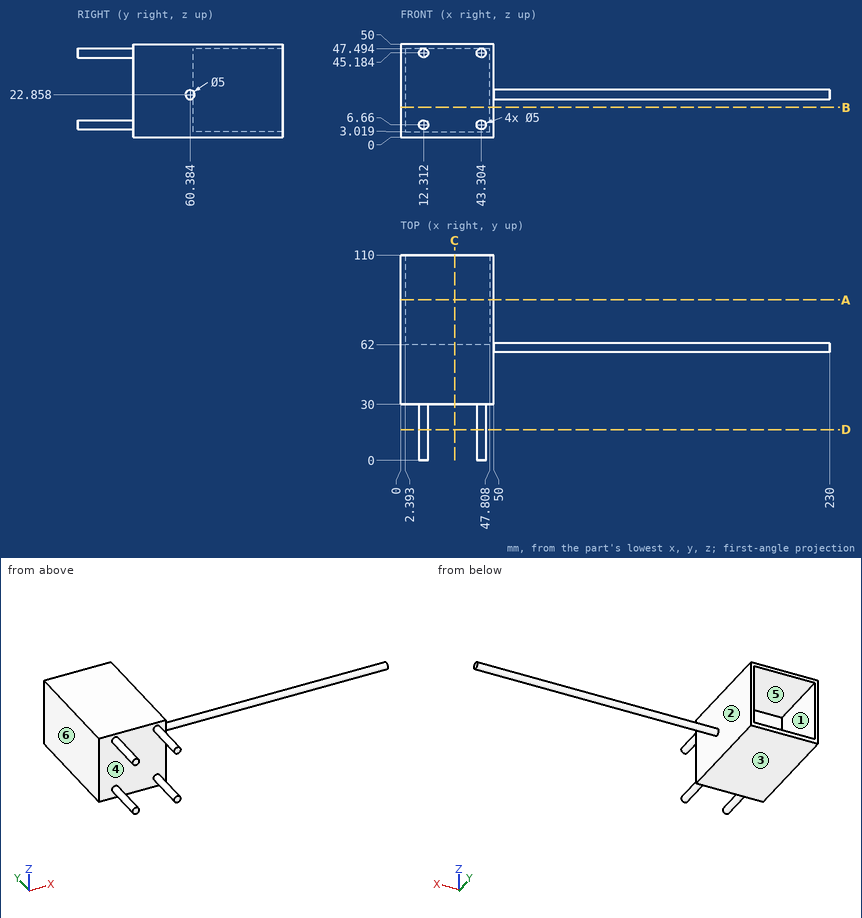
Study the drawing (mm; zero at the part's minimum x, y, z) and answer. A direction names the side the tool comes from. Round coordinates to 2 decimals unless told otherwise and drop trailing zeros. Write each loop counter-clockwise with the first axis right and the second up, starting at its lowest first coordinate (ties: lowest second). Pieces come first, ordered by that corner, then holes. Notation, with made-up numbers: (17.25, -32) -> (69.25, -32) arc R12 cw to (69.25, -17) -> close; hole circle Ø2 at (2.25, 72.25). An arc over 180 degrees is marked (long way). Answer as CSV lines item,"result". Start each with the question number.
(1) The part is cut by section C-C, the plane x = 29. Give the vertices of the cut face in (y, z) (1 decimal).
(2) Each of these flat-tipped pins is pushed along its axis until it touches: pin 1 (4 mm diameter, centred on x = 172.5, z = 21, fed in from -Y); pin 2 (13.5 mm diameter, centred on x = 22.5, y = 84, fed in from -Z); pin 3 (10 mm diameter, centred on y = 12.5, z = 5.5, fed in from +X) (1 decimal); pin 4 (22 mm diameter, centred on x = 33.5, z = 33.5, fed in from +Y). Where does it stop, or does it pass through?
(3) The part is cut by section A-A, the plane y = 86. Give the vertices of the cut face in (x, z) (1 decimal).
(4) A tool of negligible diameter and unlimited length cuts with its end or side. For the marked faces 4, 5 and 6, from which of +Z, -Z, +X, -X, +Y, -Y can it reach the whole face along a straight path? Write none if from no direction.
(5) The part is cut by section D-D, the plane y = 16.5. Give the vertices of the cut face in (x, z) (1 decimal).
(6) The mould has two halves that part along X. Classify the marked faces 1, 2 and 3: +X half, -X half, draft (parallel to the pull), parting line (faces both ways), or undercut.
(7) The part is cut by section B-B, the plane z = 16. Give the vertices of the cut face in (x, y).
(8) Find the intervals of material crossed by probe 1 along X at (y, z) = (98, 43); probe 2 along Z at (x, y) = (31.5, 98.5) (1 decimal); probe 3 along Y at (x, z) = (20, 18), in increasing order.
Output values:
1,outline,"(30, 0) -> (110, 0) -> (110, 3) -> (62, 3) -> (62, 47.5) -> (110, 47.5) -> (110, 50) -> (30, 50) -> close"
2,pin 1,"stops at y = 57.88"
2,pin 2,"stops at z = 0"
2,pin 3,"stops at x = 45.8"
2,pin 4,"stops at y = 62"
3,outline,"(0, 0) -> (50, 0) -> (50, 50) -> (0, 50) -> close; hole (2.4, 3) -> (47.8, 3) -> (47.8, 47.5) -> (2.4, 47.5) -> close"
4,face 4,"-Y"
4,face 5,"+Y"
4,face 6,"+Z, -Z, -X, +Y, -Y"
5,outline,"circle Ø5 at (12.3, 6.7); circle Ø5 at (12.3, 45.2); circle Ø5 at (43.3, 6.7); circle Ø5 at (43.3, 45.2)"
6,face 1,"undercut"
6,face 2,"+X half"
6,face 3,"draft"
7,outline,"(0, 30) -> (50, 30) -> (50, 110) -> (47.81, 110) -> (47.81, 62) -> (2.39, 62) -> (2.39, 110) -> (0, 110) -> close"
8,probe 1,"x = 0 to 2.39, 47.81 to 50"
8,probe 2,"z = 0 to 3, 47.5 to 50"
8,probe 3,"y = 30 to 62"
